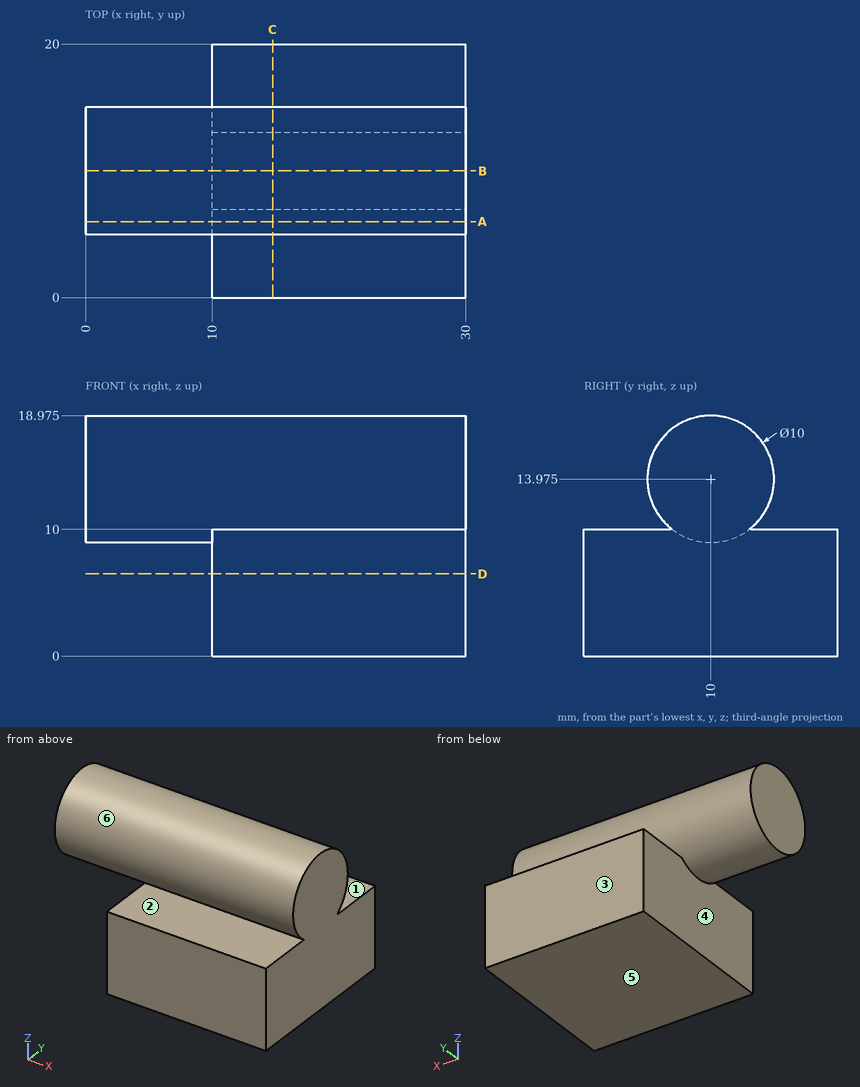
Study the drawing (mm; zero at the part's minimum x, y, z) and answer. A direction names the side the tool comes from. Give positions to 0.01 mm unless a question says otherwise; leave off trailing zeros. Order: outer loops, then holes, each group sorted by start corner. A loop starts at its lowest first (then second) coordinate and runs counter-clockwise, first axis right, second up. Notation, with made-up numbers: (-16, 62.5) - (33, 62.5) arc R25 cw to (33, 95.5) - close; hole circle Ø5 at (61.25, -38.5). An arc over 180 degrees is marked (long way). Answer as CSV lines item,"result". Start each with the question number.
Q1. For the marked faces 1, 2 and 3, determine the directions among +Z, -Z, +X, -X, +Y, -Y from which every point of the face is accessible in a straight line to the end or side of a thin tool.
Q2. The part is cut by section D-D (z = 6.5). Write down the section's boundary in (x, y), then the cut area to 3 significant figures.
Q3. The part is cut by section A-A (y = 6). Write down the section's boundary in (x, z) (1 decimal).
Q4. The part is cut by section C-C (x = 14.75). Write down the section's boundary in (y, z) (1 decimal), then the cut area to 3 significant figures.
Q5. The part is cut by section B-B (y = 10). Write down the section's boundary in (x, z) (1 decimal).
Q6. Given pin 1 Ø1 at (x, y) = (16.5, 7) entering from +Z (1 decimal); pin 2 Ø5 at (y, z) = (9.5, 5) entering from -X; pin 3 Ø5 at (x, y) = (4, 10) entering from -Z (3 decimals), each flat-ended and moving along its own axis, determine where each tip first touches the part or whether it passes through.
Q7. Find the intervals of material crossed by L1, parallel to Z at x = 15, y = 18.25; L2, parallel to X at y = 1.25, z = 6.75; L3, parallel to Z at x = 22.75, y = 12.75, in increasing order. Write a range as [from, to].
Q8. The mould has two halves that part along Z. Classify the marked faces 4, 5 and 6: +Z half, -Z half, draft (parallel to the pull), parting line (faces both ways), or undercut.
Check result:
1,face 1,"+X, -X, +Y"
1,face 2,"+X, -X, -Y"
1,face 3,"+Z, -Z, +X, -X, +Y"
2,outline,"(10, 0) - (30, 0) - (30, 20) - (10, 20) - close"
2,area,"400 mm²"
3,outline,"(0, 11) - (30, 11) - (30, 17) - (0, 17) - close; (10, 0) - (30, 0) - (30, 10) - (10, 10) - close"
4,outline,"(0, 0) - (20, 0) - (20, 10) - (13, 10) arc R5 ccw (long way) to (7, 10) - (0, 10) - close"
4,area,"274 mm²"
5,outline,"(0, 9) - (10, 9) - (10, 0) - (30, 0) - (30, 19) - (0, 19) - close"
6,pin 1,"stops at z = 18.3"
6,pin 2,"stops at x = 10"
6,pin 3,"stops at z = 8.975"
7,L1,"z = [0, 10]"
7,L2,"x = [10, 30]"
7,L3,"z = [0, 18.15]"
8,face 4,"draft"
8,face 5,"-Z half"
8,face 6,"undercut"
